```python
from build123d import *

# Parameters (mm, degrees)
SKETCH1_R           = 16
BOSS_EXTRUDE1_DEPTH = 5
SKETCH2_R           = 6.5
CUT_EXTRUDE2_DEPTH  = 2
SKETCH3_R           = 1
CUT_EXTRUDE3_DEPTH  = 3
SKETCH4_R           = 1.2
CUT_EXTRUDE4_DEPTH  = 3
SKETCH6_R           = 1
CUT_EXTRUDE6_DEPTH  = 3
CIRPATTERN3_COUNT   = 6
CIRPATTERN5_COUNT   = 6


with BuildPart() as part:
    # Sketch1 → Boss-Extrude1 (new body)
    with BuildSketch(Plane(origin=(0, 0, 0), x_dir=(1, 0, 0), z_dir=(0, 1, 0))):
        Circle(SKETCH1_R)
    extrude(amount=BOSS_EXTRUDE1_DEPTH)

    # Sketch2 → Cut-Extrude2 (cut)
    with BuildSketch(Plane(origin=(0, 5, 0), x_dir=(1, 0, 0), z_dir=(0, 1, 0))):
        Circle(SKETCH2_R)
    extrude(amount=-CUT_EXTRUDE2_DEPTH, mode=Mode.SUBTRACT)

    # Sketch3 → Cut-Extrude3 (cut)
    with BuildSketch(Plane(origin=(0, 3, 0), x_dir=(1, 0, 0), z_dir=(0, 1, 0))):
        Circle(SKETCH3_R)
    extrude(amount=-CUT_EXTRUDE3_DEPTH, mode=Mode.SUBTRACT)

    # Sketch4 → Cut-Extrude4 (cut)
    with BuildSketch(Plane(origin=(0, 3, 0), x_dir=(1, 0, 0), z_dir=(0, 1, 0))):
        with Locations((3.2, 0)):
            Circle(SKETCH4_R)
    cut_extrude4 = extrude(amount=-CUT_EXTRUDE4_DEPTH, mode=Mode.SUBTRACT)

    # Sketch6 → Cut-Extrude6 (cut)
    with BuildSketch(Plane(origin=(0, 3, 0), x_dir=(1, 0, 0), z_dir=(0, 1, 0))):
        with Locations((0, 5)):
            Circle(SKETCH6_R)
    cut_extrude6 = extrude(amount=-CUT_EXTRUDE6_DEPTH, mode=Mode.SUBTRACT)

    # CirPattern3: Cut-Extrude6 ×6 about axis
    cirpattern3_axis = Axis((0, 0, 0), (0, 1, 0))
    for i in range(1, CIRPATTERN3_COUNT):
        add(cut_extrude6.rotate(cirpattern3_axis, i * 360 / CIRPATTERN3_COUNT), mode=Mode.SUBTRACT)

    # CirPattern5: Cut-Extrude4 ×6 about axis
    cirpattern5_axis = Axis((0, 0, 0), (0, 1, 0))
    for i in range(1, CIRPATTERN5_COUNT):
        add(cut_extrude4.rotate(cirpattern5_axis, i * 360 / CIRPATTERN5_COUNT), mode=Mode.SUBTRACT)


solid = part.part
```
Build history of the part. All positions in model axes, mm. A direction names the side the tool comes from. Give positions to 0.01 mm unless a question says otherwise; leave off trailing zeros. Loops run counter-clockwise (first coordinate to the right, second up) from the corner with the lowest first, then second, coordinate; pieces in that order, holes last. Notation, with made-up numbers: (50, -16) -> (108, -16) arc R32 ccw to (108, 15) -> close; hole circle Ø1 at (15, -34.75). An arc over 180 degrees is marked (long way). One line per question, with ' | ' between items. Start each with the question number.
1) Two-plate mould, pull along Z, no slides. Class faces 3 (the cylindrical face through (-3.47, 2.46, 15.62)), 4 (the flat face through (7, 5, 0)), 5 (the cylindrical face through (-1.76, 1.52, 1.58)): released by +Z, released by -Z, zero draft, split by the parting line, or undercut.
2) Cut at D-D (y = 1.6). Count the separate pieces of the cut face and the enclosed holes in it, plus the area to 3 significant figures.
3) Cut at C-C (x = 1.6). Give the cut face in (y, z), plus the area to 3 significant figures.
4) Cut at B-B (z = 5). Give the cut face in (x, y).
5) Pin check, flat tip, straight feed: pin 1 (5 mm diameter, centred on x = 1.5, z = -0.5, fed in from +Y). Stop position of the tip, or through.
6) Cut at A-A (z = 0). Give the cut face in (x, y), plus the area to 3 significant figures.
7) 3-axis set-ups, long thin cutter, end or side, ignore diameter. For faces 1 (the cylindrical face through (-3.376, 1.521, 2.2)), 2 (the cylindrical face through (-5.158, 4.014, 3.955)): which of +Z, -Z, +X, -X, +Y, -Y reach the whole face in a straight line?
8) Probe L1, parallel to Z at x = 0, y = 0.75; L2, parallel to Z at x = 6, y = 4.75; L3, parallel to Z at x = -3.2, y = 2.25. List the from-to ranges inside material, lowest first.
Return value:
1) face 3: split by the parting line | face 4: zero draft | face 5: undercut
2) separate pieces: 1 | enclosed holes: 13 | area: 755 mm^2
3) outline: (0, -15.92) -> (5, -15.92) -> (5, -6.3) -> (3, -6.3) -> (3, -3.97) -> (0, -3.97) -> close; (0, -1.57) -> (3, -1.57) -> (3, 1.57) -> (0, 1.57) -> close; (0, 3.97) -> (3, 3.97) -> (3, 6.3) -> (5, 6.3) -> (5, 15.92) -> (0, 15.92) -> close | area: 120 mm^2
4) outline: (-15.2, 0) -> (-1, 0) -> (-1, 3) -> (-4.15, 3) -> (-4.15, 5) -> (-15.2, 5) -> close; (1, 0) -> (15.2, 0) -> (15.2, 5) -> (4.15, 5) -> (4.15, 3) -> (1, 3) -> close
5) pin 1: y = 3
6) outline: (-16, 0) -> (-4.4, 0) -> (-4.4, 3) -> (-6.5, 3) -> (-6.5, 5) -> (-16, 5) -> close; (-2, 0) -> (-1, 0) -> (-1, 3) -> (-2, 3) -> close; (1, 0) -> (2, 0) -> (2, 3) -> (1, 3) -> close; (4.4, 0) -> (16, 0) -> (16, 5) -> (6.5, 5) -> (6.5, 3) -> (4.4, 3) -> close | area: 114 mm^2
7) face 1: +Y, -Y | face 2: +Y
8) L1: -16 to -6, -4 to -1, 1 to 4, 6 to 16 | L2: -14.83 to -2.5, 2.5 to 14.83 | L3: -15.68 to -1.2, 1.2 to 15.68
